Geometry: final body of the model. Coordinates: model frame, mm. Face numbers are marked on the shaded views. A direction names the side the tool comes from. Give positions to 0.01 mm unless a question says otherwise; leave off trailing zeros. Loops run counter-clockwise (first coordinate to the right, second up) from the corner with the lowest first, then second, coordinate; pieces in that order, holes last. Notation, with made-up numbers: (35, 86) -> (72, 86) arc R28 ccw to (72, 110) -> close; hole circle Ø4 at (6.25, 7.25). An arc over 180 degrees is marked (long way). One line per item, written item: value. Start each with the question number.
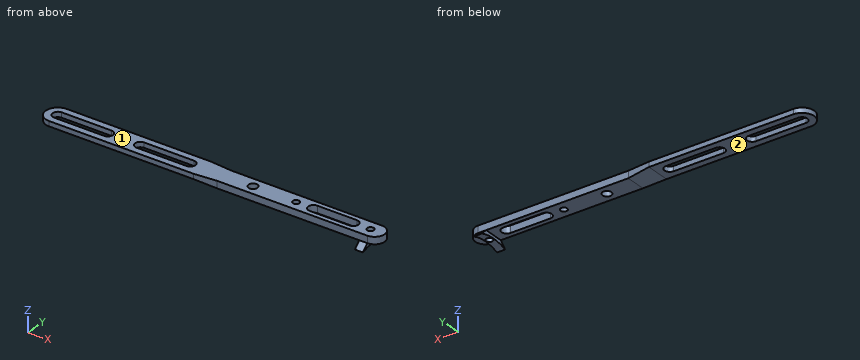
from build123d import *

# Parameters (mm, degrees)
F0_R      = 1.65
F1_DEPTH  = 3.5
F3_DEPTH  = 6
F6_DEPTH  = 2
F9_DEPTH  = 1.75
F11_D     = 4.5
F11_DEPTH = 52.4
F11_TIP   = 1.3519363928


# Not quite as in the source:
# - a feature names something its author has since deleted; it is built from what else it names


with BuildPart() as f1:
    # F0 (on Top) → F1 (new body)
    with BuildSketch(Plane.XY):
        with BuildLine():
            Line((0, 6), (-71.8000936901, 6))
            ThreePointArc((-71.8000936901, 6), (-77.8000936901, 0), (-71.8000936901, -6))
            Line((-71.8000936901, -6), (0, -6))
            Line((0, -6), (11, -5))
            Line((11, -5), (85.6788979987, -5))
            ThreePointArc((85.6788979733, -4.9999999898), (90.6788979733, 3.56e-08), (85.6788979225, 5.0000000102))
            Line((85.6788979479, 5.0000000203), (11, 4.9999992617))
            Line((11, 4.9999992617), (0, 6))
        make_face()
        with Locations((46.6788982548, -0.0513669582)):
            Circle(F0_R, mode=Mode.SUBTRACT)
        with BuildLine():
            ThreePointArc((75.0788576977, 2.5999999997), (77.6788979986, 1.85129e-05), (75.0788947235, -2.6))
            Line((75.0788947235, -2.6), (55.290283107, -2.5999750728))
            ThreePointArc((55.290283107, -2.5999750728), (55.2788947235, -2.6), (55.2675063401, -2.5999750441))
            ThreePointArc((55.2675063401, -2.5999750441), (52.6790245248, 0.02564995), (55.3188054687, 2.5996937115))
            Line((55.3188054687, 2.5996937115), (75.0788576977, 2.5999999997))
        make_face(mode=Mode.SUBTRACT)
        with BuildLine():
            ThreePointArc((-71.8000936901, -2.6), (-74.4000936901, 0), (-71.8000936901, 2.6))
            Line((-71.8000936901, 2.6), (-47.0008072172, 2.6))
            ThreePointArc((-47.0008072172, 2.6), (-44.4008072172, 0), (-47.0008072172, -2.6))
            Line((-47.0008072172, -2.6), (-71.8000936901, -2.6))
        make_face(mode=Mode.SUBTRACT)
        with BuildLine():
            ThreePointArc((-30.8000002499, -2.6), (-33.4000002499, 0), (-30.8000002499, 2.6))
            Line((-30.8000002499, 2.6), (-6.00000025, 2.6))
            ThreePointArc((-6.00000025, 2.6), (-5.9984911006, 2.599999562), (-5.9969819517, 2.5999982481))
            ThreePointArc((-5.9969819517, 2.5999982481), (-3.400000688, -0.0015091494), (-6.00000025, -2.6))
            Line((-6.00000025, -2.6), (-30.8000002499, -2.6))
        make_face(mode=Mode.SUBTRACT)
        with Locations((83.6788979987, 0)):
            Circle(F0_R, mode=Mode.SUBTRACT)
    extrude(amount=F1_DEPTH)

    # F2 (on Front) → F3 (cut, symmetric)
    with BuildSketch(Plane.XZ):
        Polygon((-80.4351404223, 1), (-80.4351404223, 0), (11, 0), (0, 1), align=None)
    extrude(amount=F3_DEPTH, both=True, mode=Mode.SUBTRACT)

    # F5 (on face) → F6 (join, symmetric)
    with BuildSketch(Plane.YZ.offset(83.6788979987)):
        Polygon((-5.7500000356, -0.75), (5.7500000356, -0.75), (5.0000000356, 0), (-5.0000000356, 0), align=None)
        with BuildLine():
            ThreePointArc((-7.9520996302, -2.9520995947), (0, -1.5), (7.9520996302, -2.9520995946))
            Line((7.9520996302, -2.9520995946), (5.7500000356, -0.75))
            Line((5.7500000356, -0.75), (-5.7500000356, -0.75))
            Line((-5.7500000356, -0.75), (-7.9520996302, -2.9520995946))
        make_face()
    extrude(amount=F6_DEPTH, both=True)

    # F9 (cut): a face of the model
    f9_faces = [f1.faces().sort_by_distance(p)[0] for p in [
        (83.6788979987, 0, 0),
    ]]
    extrude(f9_faces, amount=-F9_DEPTH, mode=Mode.SUBTRACT)

    # F11
    with Locations(Plane.XY.offset(3.5)):
        with Locations((25.2248030156, 0)):
            Hole(F11_D / 2, depth=F11_DEPTH)
            with Locations((0, 0, -(F11_DEPTH + F11_TIP / 2))):  # 118° drill point
                Cone(0, F11_D / 2, F11_TIP, mode=Mode.SUBTRACT)


solid = f1.part
Item 1: Pin query (flat end, axial travel): pin 1 (1.8 mm diameter, centred on x = 57.5, z = 1, fed in from +Y); pin 2 (1.2 mm diameter, centred on x = -56.5, z = 1.5, fed in from -Y); pin 3 (3.5 mm diameter, centred on x = -57.5, y = 1.5, fed in from -Z). Return the tip coordinate at first contact, or that it passes through.
Item 2: Access query for the marked faces 1 and 2. Directions: +Z, -Z, +X, -X, +Y, -Y. A direction counts if a zero-diameter tool reaches every point of the face in a straight line with its end or side. Return the directions, or none.
Item 3: Ray query, line 1 along X through (y, z) = (0, -0.5); line 2 along Z through (x, y) = (74.5, 2.75); line 3 along X through (y, z) = (6.75, -2.5). Return the intervals inside material, ascending. Write a range as [from, to].
Item 4: Section B-B, the plane z = 2.25. State how many separate pieces and enclosed holes the cut face has, then the cut area to 3 significant figures.
Item 5: Section A-A, the plane x = -19. Output: boundary loops of the cut face in (y, z).
Geometry check:
1. pin 1: stops at y = 5
1. pin 2: stops at y = -6
1. pin 3: stops at z = 1
2. face 1: +Z, +X, -X, +Y, -Y
2. face 2: -Z, -X, +Y, -Y
3. line 1: x = [81.68, 82.03], [85.33, 85.68]
3. line 2: z = [0, 3.5]
3. line 3: x = [81.68, 85.68]
4. separate pieces: 1
4. enclosed holes: 6
4. area: 1,370 mm2
5. outline: (-6, 1) -> (-2.6, 1) -> (-2.6, 3.5) -> (-6, 3.5) -> close; (2.6, 1) -> (6, 1) -> (6, 3.5) -> (2.6, 3.5) -> close
